```python
from build123d import *

# Parameters (mm, degrees)
SKETCH1_R           = 5
BOSS_EXTRUDE1_DEPTH = 10
SKETCH2_R           = 2
CUT_EXTRUDE1_DEPTH  = 10
CUT_EXTRUDE2_DEPTH  = 24
CHAMFER1_SIZE       = 1


with BuildPart() as part:
    # Sketch1 → Boss-Extrude1 (new body)
    with BuildSketch(Plane(origin=(0, 0, 0), x_dir=(0, 0, -1), z_dir=(1, 0, 0))):
        with BuildLine():
            Line((-18, 30.175), (-18, 0))
            Line((-18, 0), (0, 0))
            Line((0, 0), (0, 30.175))
            ThreePointArc((0, 30.175), (-9, 39.175), (-18, 30.175))
        make_face()
        with Locations((-9, 30.175)):
            Circle(SKETCH1_R, mode=Mode.SUBTRACT)
    extrude(amount=BOSS_EXTRUDE1_DEPTH)

    # Sketch2 → Cut-Extrude1 (cut)
    with BuildSketch(Plane.XZ):
        with Locations(Location((5, 4, 0), (0, 0, 270))):
            Circle(SKETCH2_R)
        with Locations(Location((5, 14, 0), (0, 0, 270))):
            Circle(SKETCH2_R)
    extrude(amount=-CUT_EXTRUDE1_DEPTH, mode=Mode.SUBTRACT)

    # Sketch3 → Cut-Extrude2 (cut)
    with BuildSketch(Plane.XY):
        Polygon((10, 6.35), (6.35, 14.17745026), (6.35, 39.175), (10, 39.175), align=None)
    extrude(amount=CUT_EXTRUDE2_DEPTH, mode=Mode.SUBTRACT)

    # Chamfer1
    chamfer1_edges = [part.edges().sort_by_distance(p)[0] for p in [
        (10, 3.175, 0),
        (10, 3.175, 18),
        (8.175, 10.26372513, 0),
        (6.35, 22.17622513, 0),
        (6.35, 39.175, 9),
        (6.35, 22.17622513, 18),
        (8.175, 10.26372513, 18),
        (0, 15.0875, 0),
        (0, 15.0875, 18),
        (0, 39.175, 9),
    ]]
    chamfer(chamfer1_edges, length=CHAMFER1_SIZE)


solid = part.part
```
Source: CAD feature listing. Evaluate the final solid. Frame: model axes, mm. A direction names the side the tool comes from. Round coordinates to 2 decimals unless told otherwise and drop trailing zeros. Order: outer loops, then holes, each group sorted by start corner. A loop starts at its lowest first (then second) coordinate and runs counter-clockwise, first axis right, second up. Notation, with made-up numbers: (44, 66) -> (74, 66) arc R9 cw to (74, 73) -> close; hole circle Ø8 at (5.5, 74). An arc over 180 degrees is marked (long way). Use CSV: the item, a comma, the result in double quotes.
(1) Pull-direction query (X, two-part tool) for faces 1 (the face through (7, 5, 14)), 2 (the face through (5.86, 21.95, 0.51)), 3 (the face through (0, 15, 9)); classes: +X half, -X half, draft (parallel to the pull), parting line (faces both ways), or undercut.
Report:
face 1,"undercut"
face 2,"+X half"
face 3,"-X half"
(2) First-contact query: pin 1 Ø5 at (y, z) = (25, 7) entering from +X; pin 2 Ø1.5 at (x, z) = (3.5, 14) entering from +Y; pin 3 Ø6 at (x, z) = (2, 5.5) entering from +Y. Flat tips, straight axial feed; report the tip coordinate or a pass-through.
Report:
pin 1,"x = 6.35"
pin 2,"y = 38.11"
pin 3,"y = 39.16"
(3) Section C-C on x = 3.5. Return the cut outline in (y, z) (3 decimals), and give its area (3 significant figures).
Report:
outline,"(0, 0) -> (30.175, 0) arc R9 ccw to (30.175, 18) -> (0, 18) -> (0, 15.323) -> (10, 15.323) -> (10, 12.677) -> (0, 12.677) -> (0, 5.323) -> (10, 5.323) -> (10, 2.677) -> (0, 2.677) -> close; hole circle Ø10 at (30.175, 9)"
area,"539 mm^2"
(4) Section A-A on z = 9. Return the cut outline in (x, y) (3 decimals), and give its area (3 significant figures).
Report:
outline,"(0, 0) -> (10, 0) -> (10, 6.35) -> (6.35, 14.177) -> (6.35, 25.175) -> (0, 25.175) -> close; (0, 35.175) -> (6.35, 35.175) -> (6.35, 38.175) -> (5.35, 39.175) -> (1, 39.175) -> (0, 38.175) -> close"
area,"222 mm^2"
(5) Access query for faces 4 (the face through (5, 10, 4)), 5 (the face through (6.35, 23, 9)), 6 (the face through (5.86, 22.18, 17.49)). Directions: +Z, -Z, +X, -X, +Y, -Y. A direction counts if a zero-diameter tool reaches every point of the face in a straight line with its end or side. Return the directions, or none.
Report:
face 4,"-Y"
face 5,"+Z, -Z, +X, +Y"
face 6,"+Z, +X, +Y"
(6) Section D-D on x = 8. Return the cut outline in (y, z), and give its area (3 significant figures).
Report:
outline,"(0, 0) -> (8.27, 0) -> (10.64, 1) -> (10.64, 17) -> (8.27, 18) -> (0, 18) -> close"
area,"189 mm^2"
(7) Ray query, L1, parallel to Y at x = 5, z = 9 (3 decimals); L2, parallel to X at y = 2.5, z = 4; L3, parallel to X at y = 18.5, z = 8. Return the intervals inside material, ascending.
Report:
L1,"0 to 25.175, 35.175 to 39.175"
L2,"0 to 3, 7 to 10"
L3,"0 to 6.35"
(8) Section B-B on y = 27. Return the cut outline in (x, z).
Report:
outline,"(0, 1) -> (1, 0) -> (5.35, 0) -> (6.35, 1) -> (6.35, 5.14) -> (0, 5.14) -> close; (0, 12.86) -> (6.35, 12.86) -> (6.35, 17) -> (5.35, 18) -> (1, 18) -> (0, 17) -> close"
